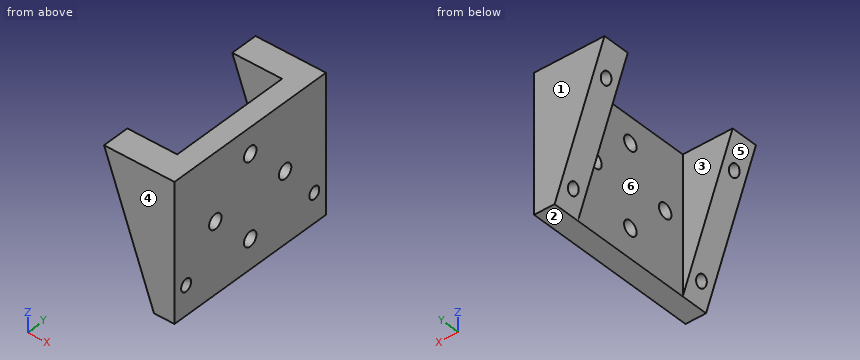
from build123d import *

# Parameters (mm, degrees)
BOSS_EXTRUDE1_DEPTH       = 20.6375
M3_CLEARANCE_HOLE1_D      = 3.4
CUT_EXTRUDE1_DEPTH        = 14.2875
CUT_EXTRUDE1_DEPTH_BACK   = 14.2875
F_6_32_TAPPED_HOLE1_D     = 2.7051
F_6_32_TAPPED_HOLE1_DEPTH = 8.382
F_6_32_TAPPED_HOLE1_TIP   = 0.81269403


with BuildPart() as part:
    # Sketch1 → Boss-Extrude1 (new body, symmetric)
    with BuildSketch(Plane(origin=(0, 0, 0), x_dir=(1, 0, 0), z_dir=(0, 1, 0))):
        Polygon((0, 0), (-11.556054938, -31.75), (4.7625, -31.75), (4.7625, 0), align=None)
    extrude(amount=BOSS_EXTRUDE1_DEPTH, both=True)

    # M3 Clearance Hole1 (through all)
    with Locations(Plane(origin=(4.7625, 0, 0), x_dir=(0, 0, -1), z_dir=(1, 0, 0))):
        with Locations((-16.3125, 9.5), (-6.8125, 0), (-16.3125, -9.5), (-25.8125, 0)):
            Hole(M3_CLEARANCE_HOLE1_D / 2)

    # Sketch15 → Cut-Extrude1 (cut, two sides)
    with BuildSketch(Plane(origin=(0, 0, 0), x_dir=(1, 0, 0), z_dir=(0, 1, 0))) as cut_extrude1_sk:
        Polygon((-11.556054938, -31.75), (0, 0), (0, -31.75), align=None)
    extrude(amount=CUT_EXTRUDE1_DEPTH, mode=Mode.SUBTRACT)
    extrude(cut_extrude1_sk.sketch, amount=-CUT_EXTRUDE1_DEPTH_BACK, mode=Mode.SUBTRACT)

    # #6-32 Tapped Hole1
    with Locations(Plane(origin=(0, 0, 0), x_dir=(-0.342020143, 0, 0.939692621), z_dir=(-0.939692621, 0, -0.342020143))):
        with Locations((4.7625, 17.4625), (26.9875, 17.4625), (26.9875, -17.4625), (4.7625, -17.4625)):
            Hole(F_6_32_TAPPED_HOLE1_D / 2, depth=F_6_32_TAPPED_HOLE1_DEPTH)
            with Locations((0, 0, -(F_6_32_TAPPED_HOLE1_DEPTH + F_6_32_TAPPED_HOLE1_TIP / 2))):  # 118° drill point
                Cone(0, F_6_32_TAPPED_HOLE1_D / 2, F_6_32_TAPPED_HOLE1_TIP, mode=Mode.SUBTRACT)


solid = part.part
The listing builds one solid part. Answer for the finished solid, in the listing's coordinates (mm). Face numbers are marked on the shaded views. A direction names the side the tool comes from. Coordinates: 2 decimals unless noted, no trailing zeros. Write each loop counter-clockwise with the first axis right and the second up, starting at its lowest first coordinate (ties: lowest second). Pieces come first, ordered by that corner, then holes. Notation, with made-up numbers: (-7, -30) - (25, -30) arc R27 ccw to (25, 4) - close; hole circle Ø5 at (-26.75, 47.5). An arc over 180 degrees is marked (long way). Put each result on its own line as item: value.
1. Flat-ended cylindrical pins translate along their axes: pin 1 Ø1.5 at (x, z) = (-10, 25.5) entering from +Y; pin 2 Ø2 at (y, z) = (15.5, 21.5) entering from -X; pin 3 Ø5.5 at (y, z) = (9.5, 16.31) entering from -X. Find the tip coordinate at first contact, or state that the pin passes through.
Answer sheet:
pin 1: stops at y = 20.64
pin 2: stops at x = -8.19
pin 3: stops at x = 0
2. The part is cut by section B-B on y = -9.5. Give the vertices of the cut face in (x, z), plus the area to 3 significant figures.
Answer sheet:
outline: (0, 0) - (4.76, 0) - (4.76, 14.61) - (0, 14.61) - close; (0, 18.01) - (4.76, 18.01) - (4.76, 31.75) - (0, 31.75) - close
area: 135 mm^2
3. Determine the mould class of the marked faces 1, 2, 3 and 4 for opening direction Y: pulls with the +Y half, pulls with the -Y half, needs draft (parallel to the pull), parting line crosses it, or undercut.
Answer sheet:
face 1: pulls with the +Y half
face 2: needs draft
face 3: undercut
face 4: pulls with the -Y half
4. The part is cut by section D-D on x = 2.25. State how many separate pieces and enclosed holes the cut face has, plus the area to 3 significant figures.
Answer sheet:
separate pieces: 1
enclosed holes: 6
area: 1,260 mm^2
5. The part is cut by section C-C on z = 16.5. Give the vertices of the cut face in (x, y), plus the area to 3 significant figures.
Answer sheet:
outline: (-6.01, -20.64) - (4.76, -20.64) - (4.76, -11.19) - (0, -11.19) - (0, -14.29) - (-6.01, -14.29) - close; (-6.01, 14.29) - (0, 14.29) - (0, 11.19) - (4.76, 11.19) - (4.76, 20.64) - (-6.01, 20.64) - close; (0, -7.81) - (4.76, -7.81) - (4.76, 7.81) - (0, 7.81) - close
area: 241 mm^2
6. Find the intervals of material crossed by line 1 along Z through (x, y) = (1.15, 0); line 2 along Y through (x, z) = (-3.25, 23); line 3 along Y through (x, z) = (-0.75, 3.5), in increasing order. Write a range as from..to.
Answer sheet:
line 1: z = 0..5.11, 8.51..24.11, 27.51..31.75
line 2: y = -20.64..-14.29, 14.29..20.64
line 3: y = -20.64..-18.05, -16.87..-14.29, 14.29..16.87, 18.05..20.64
7. A tool of negligible diameter and unlimited length cuts with its end or side. For the marked faces 5 and 6, from which of +Z, -Z, +X, -X, +Y, -Y can it reach the whole face along a straight path? Write none if from no direction.
Answer sheet:
face 5: -Z, -X, +Y, -Y
face 6: +Z, -Z, -X
8. The part is cut by section A-A on y = 0. Give the vertices of the cut face in (x, z), plus the area to 3 significant figures.
Answer sheet:
outline: (0, 0) - (4.76, 0) - (4.76, 5.11) - (0, 5.11) - close; (0, 8.51) - (4.76, 8.51) - (4.76, 24.11) - (0, 24.11) - close; (0, 27.51) - (4.76, 27.51) - (4.76, 31.75) - (0, 31.75) - close
area: 119 mm^2
